Geometry check sheet. Reference: the model listing, model coordinates, mm. A direction names the side the tool comes from. Give positions to 0.01 mm unless a question says otherwise; leave off trailing zeros. Write each loop counter-clockwise with the first axis right and the second up, starting at its lowest first coordinate (ties: lowest second). Pieces come first, ordered by that corner, then holes. Notation, with made-up numbers: M -40,48 L -3,48 A19 ccw -3,74 Z; hole C -14.5,49.5 d5. An arc over 180 degrees is marked long. One line per item, written item: value. Start each with the question number.
1. Cross-section at C-C on z = 28.5. Record the cut outline in (x, y), then the cut area to 3 significant figures.
2. Cross-section at A-A on x = -106. Record the cut outline in (y, z).
3. Release check for a two-part mould opening along Y. For faces 5 (the face through (-32, 101.6, 8)), 6 (the face through (-0.864, 232, 20)), 7 (the face through (-89, 156, 1.575)) record: pulls with the +Y half, pulls with the -Y half, needs draft (parallel to the pull), parting line crosses it, or undercut.
4. Cross-section at D-D on x = -241. Record the cut outline in (y, z).
5. Gauge pin test, flat ends, axial feed: pin 1 (4 mm diameter, centred on x = -163.83, y = 78.74, fed in from +Z); pin 2 (2 mm diameter, centred on x = -234.5, y = 110, fed in from -Z); pin 3 (1.5 mm diameter, centred on x = -257, z = 6.5, fed in from +Y); pin 4 (7.5 mm diameter, centred on y = 230.5, z = 18.5, fed in from +X). Record the tip position at first contact, or that the pin passes through.
6. Tool access check on faces 1 (the face through (-184, 44.45, 8)), 2 (the face through (-247.943, 33.657, 7.836)), 3 (the face through (-44.45, 139, 8)), 4 (the face through (-78, 219.583, 20)). Record the directions out of +Z, -Z, +X, -X, +Y, -Y that give a thin tool (end or side, any length) a straight path to the whole face; none if there is none.
7. Scan lines: line 1 (Y direction, x = -288.29, z = 0.55); line 2 (Y direction, x = -88.9, z = 7.75) (3 decimals); line 3 (X direction, y = 233.68, z = 0.35). Record each from-to range of solid material in increasing order.
8. Cross-section at B-B on y = 57.15. Record the cut outline in (x, z).
from build123d import *

# Parameters (mm, degrees)
F0_W     = 304.8
F0_H     = 243.84
F0_R     = 2.0955
F1_DEPTH = 1.5748
F2_W     = 152.146
F2_H     = 25.4
F3_DEPTH = 37.338
F4_W     = 50.8
F4_H     = 50.8
F4_R     = 6.35
F5_DEPTH = 12.7
F6_W     = 25.4
F6_H     = 76.2
F6_R     = 6.35
F7_DEPTH = 12.7
F8_R     = 6.35
F9_DEPTH = 12.7


with BuildPart() as f1:
    # F0 (on Top) → F1 (new body)
    with BuildSketch(Plane.XY):
        with Locations((-152.4, 121.92)):
            Rectangle(F0_W, F0_H)
        with Locations((-288.29, 6.35)):
            Circle(F0_R, mode=Mode.SUBTRACT)
        with Locations((-163.83, 6.35)):
            Circle(F0_R, mode=Mode.SUBTRACT)
        with Locations((-288.29, 78.74)):
            Circle(F0_R, mode=Mode.SUBTRACT)
        with Locations((-163.83, 78.74)):
            Circle(F0_R, mode=Mode.SUBTRACT)
        with Locations((-6.35, 6.35)):
            Circle(F0_R, mode=Mode.SUBTRACT)
        with Locations((-6.35, 78.74)):
            Circle(F0_R, mode=Mode.SUBTRACT)
        with Locations((-288.29, 233.68)):
            Circle(F0_R, mode=Mode.SUBTRACT)
        with Locations((-209.55, 233.68)):
            Circle(F0_R, mode=Mode.SUBTRACT)
        with Locations((-163.83, 233.68)):
            Circle(F0_R, mode=Mode.SUBTRACT)
        with Locations((-6.35, 210.82)):
            Circle(F0_R, mode=Mode.SUBTRACT)
    extrude(amount=F1_DEPTH)

    # F2 (on face) → F3 (join)
    with BuildSketch(Plane.XY.offset(1.5748)):
        with Locations((-76.9366, 232.283)):
            Rectangle(F2_W, F2_H)
    extrude(amount=F3_DEPTH)

    # F4 (on face) → F5 (join)
    with BuildSketch(Plane.XY.offset(1.5748)):
        with Locations((-88.9, 139.7)):
            Rectangle(F4_W, F4_H)
        with Locations((-88.9, 123.825)):
            Circle(F4_R, mode=Mode.SUBTRACT)
        with Locations((-88.9, 155.575)):
            Circle(F4_R, mode=Mode.SUBTRACT)
    extrude(amount=F5_DEPTH)

    # F6 (on face) → F7 (join)
    with BuildSketch(Plane.XY.offset(1.5748)):
        with Locations((-31.75, 139.7)):
            Rectangle(F6_W, F6_H)
        with Locations((-31.75, 114.3)):
            Circle(F6_R, mode=Mode.SUBTRACT)
        with Locations((-31.75, 165.1)):
            Circle(F6_R, mode=Mode.SUBTRACT)
    extrude(amount=F7_DEPTH)

    # F8 (on face) → F9 (join)
    with BuildSketch(Plane.XY.offset(1.5748)):
        Polygon((-165.1, 69.85), (-266.7, 69.85), (-266.7, 19.05), (-203.2, 19.05), (-203.2, 44.45), (-165.1, 44.45), align=None)
        with Locations((-254, 31.75)):
            Circle(F8_R, mode=Mode.SUBTRACT)
        with Locations((-177.8, 57.15)):
            Circle(F8_R, mode=Mode.SUBTRACT)
    extrude(amount=F9_DEPTH)


solid = f1.part
Report:
1. outline: M -153.01,219.58 L -0.86,219.58 L -0.86,244.98 L -153.01,244.98 Z
1. area: 3,860 mm^2
2. outline: M 0,0 L 243.84,0 L 243.84,1.57 L 244.98,1.57 L 244.98,38.91 L 219.58,38.91 L 219.58,1.57 L 165.1,1.57 L 165.1,14.27 L 114.3,14.27 L 114.3,1.57 L 0,1.57 Z
3. face 5: pulls with the -Y half
3. face 6: needs draft
3. face 7: undercut
4. outline: M 0,0 L 243.84,0 L 243.84,1.57 L 69.85,1.57 L 69.85,14.27 L 19.05,14.27 L 19.05,1.57 L 0,1.57 Z
5. pin 1: passes through
5. pin 2: stops at z = 0
5. pin 3: stops at y = 69.85
5. pin 4: stops at x = -0.86
6. face 1: +Z, +X, -Y
6. face 2: +Z
6. face 3: +Z, -Y
6. face 4: +Z, +X, -X
7. line 1: y = 0 to 4.25, 8.45 to 76.64, 80.84 to 231.58, 235.78 to 243.84
7. line 2: y = 114.3 to 117.475, 130.175 to 149.225, 161.925 to 165.1, 219.583 to 244.983
7. line 3: x = -304.8 to -290.39, -286.19 to -211.65, -207.45 to -165.93, -161.73 to 0
8. outline: M -304.8,0 L 0,0 L 0,1.57 L -165.1,1.57 L -165.1,14.27 L -171.45,14.27 L -171.45,1.57 L -184.15,1.57 L -184.15,14.27 L -266.7,14.27 L -266.7,1.57 L -304.8,1.57 Z
